from build123d import *

# Parameters (mm, degrees)
SKETCH1_R           = 1.2
BOSS_EXTRUDE1_DEPTH = 10
SKETCH3_R           = 13.5
SKETCH3_R_2         = 7.75
CUT_EXTRUDE1_DEPTH  = 1
SKETCH4_W           = 28.3
SKETCH4_H           = 8.75
CUT_EXTRUDE2_DEPTH  = 6.444
CUT_EXTRUDE3_DEPTH  = 0.1
CUT_EXTRUDE4_DEPTH  = 2


with BuildPart() as part:
    # Sketch1 → Boss-Extrude1 (new body)
    with BuildSketch(Plane(origin=(0, 0, 0), x_dir=(1, 0, 0), z_dir=(0, 1, 0))):
        with BuildLine():
            Line((-13.613846154, 16.730769231), (21.306153846, 16.730769231))
            ThreePointArc((21.306153846, 16.730769231), (23.10220507, 15.986820455), (23.846153846, 14.190769231))
            Line((23.846153846, 14.190769231), (23.846153846, -20.729230769))
            ThreePointArc((23.846153846, -20.729230769), (23.10220507, -22.525281993), (21.306153846, -23.269230769))
            Line((21.306153846, -23.269230769), (-13.613846154, -23.269230769))
            ThreePointArc((-13.613846154, -23.269230769), (-15.409897378, -22.525281993), (-16.153846154, -20.729230769))
            Line((-16.153846154, -20.729230769), (-16.153846154, 14.190769231))
            ThreePointArc((-16.153846154, 14.190769231), (-15.409897378, 15.986820455), (-13.613846154, 16.730769231))
        make_face()
        with Locations(Location((-13.613846154, 14.190769231, 0), (0, 0, 270))):
            Circle(SKETCH1_R, mode=Mode.SUBTRACT)
        with Locations(Location((21.386153846, 14.190769231, 0), (0, 0, 270))):
            Circle(SKETCH1_R, mode=Mode.SUBTRACT)
        with Locations(Location((21.386153846, -20.809230769, 0), (0, 0, 270))):
            Circle(SKETCH1_R, mode=Mode.SUBTRACT)
        with Locations(Location((-13.613846154, -20.809230769, 0), (0, 0, 270))):
            Circle(SKETCH1_R, mode=Mode.SUBTRACT)
    extrude(amount=BOSS_EXTRUDE1_DEPTH)

    # Sketch3 → Cut-Extrude1 (cut)
    with BuildSketch(Plane(origin=(0, 10, 0), x_dir=(1, 0, 0), z_dir=(0, 1, 0))):
        with Locations(Location((3.846153846, -7.269230769, 0), (0, 0, 270))):
            Circle(SKETCH3_R)
        with Locations(Location((3.846153846, -7.269230769, 0), (0, 0, 270))):
            Circle(SKETCH3_R_2, mode=Mode.SUBTRACT)
    extrude(amount=-CUT_EXTRUDE1_DEPTH, mode=Mode.SUBTRACT)

    # Sketch4 → Cut-Extrude2 (cut)
    with BuildSketch(Plane.ZY.offset(16.153846154)):
        with Locations((3.419230769, 5.092214042)):
            Rectangle(SKETCH4_W, SKETCH4_H)
    extrude(amount=-CUT_EXTRUDE2_DEPTH, mode=Mode.SUBTRACT)

    # Sketch5 → Cut-Extrude3 (cut)
    with BuildSketch(Plane(origin=(0, 10, 0), x_dir=(1, 0, 0), z_dir=(0, 1, 0))):
        Polygon((-12.625840765, 10.092905938), (-12.625840765, 8.58923838), (-8.593277769, 8.58923838), (-8.593277769, 7.290616398), (-12.625840765, 7.290616398), (-12.625840765, 5.771945506), (-15.223084728, 8.179147228), align=None)
    extrude(amount=-CUT_EXTRUDE3_DEPTH, mode=Mode.SUBTRACT)

    # Sketch6 → Cut-Extrude4 (cut)
    with BuildSketch(Plane.XZ):
        with BuildLine():
            Line((-16.153846154, 17.269230769), (-13.201846154, 17.269230769))
            ThreePointArc((-13.201846154, 17.269230769), (-11.046584685, 18.1619693), (-10.153846154, 20.317230769))
            Line((-10.153846154, 20.317230769), (-10.153846154, 23.269230769))
            Line((-10.153846154, 23.269230769), (-10.153846154, 27.06129419))
            Line((-10.153846154, 27.06129419), (-21.305262053, 27.06129419))
            Line((-21.305262053, 27.06129419), (-21.305262053, 17.269230769))
            Line((-21.305262053, 17.269230769), (-16.153846154, 17.269230769))
        make_face()
        with BuildLine():
            Line((23.846153846, 17.269230769), (20.894153846, 17.269230769))
            ThreePointArc((20.894153846, 17.269230769), (18.738892377, 18.1619693), (17.846153846, 20.317230769))
            Line((17.846153846, 20.317230769), (17.846153846, 23.269230769))
            Line((17.846153846, 23.269230769), (17.846153846, 27.06129419))
            Line((17.846153846, 27.06129419), (26.668789671, 27.06129419))
            Line((26.668789671, 27.06129419), (26.668789671, 17.269230769))
            Line((26.668789671, 17.269230769), (23.846153846, 17.269230769))
        make_face()
        with BuildLine():
            Line((-10.153846154, -16.730769231), (-10.153846154, -13.778769231))
            ThreePointArc((-10.153846154, -13.778769231), (-11.046584685, -11.623507762), (-13.201846154, -10.730769231))
            Line((-13.201846154, -10.730769231), (-16.153846154, -10.730769231))
            Line((-16.153846154, -10.730769231), (-21.305262053, -10.730769231))
            Line((-21.305262053, -10.730769231), (-21.305262053, -18.817505275))
            Line((-21.305262053, -18.817505275), (-10.153846154, -18.817505275))
            Line((-10.153846154, -18.817505275), (-10.153846154, -16.730769231))
        make_face()
        with BuildLine():
            Line((17.846153846, -16.730769231), (17.846153846, -13.778769231))
            ThreePointArc((17.846153846, -13.778769231), (18.738892377, -11.623507762), (20.894153846, -10.730769231))
            Line((20.894153846, -10.730769231), (23.846153846, -10.730769231))
            Line((23.846153846, -10.730769231), (26.668789671, -10.730769231))
            Line((26.668789671, -10.730769231), (26.668789671, -18.817505275))
            Line((26.668789671, -18.817505275), (17.846153846, -18.817505275))
            Line((17.846153846, -18.817505275), (17.846153846, -16.730769231))
        make_face()
    extrude(amount=-CUT_EXTRUDE4_DEPTH, mode=Mode.SUBTRACT)


solid = part.part
Here's how the part is built. I have some questions about the finished solid (model axes, mm). A direction names the side the tool comes from. Coordinates: 2 decimals unless noted, no trailing zeros. Write each loop counter-clockwise with the first axis right and the second up, starting at its lowest first coordinate (ties: lowest second). Pieces come first, ordered by that corner, then holes.
Item 1: If we mould it in two halves opening along Z, with no side actions, what happens to faces 1 (the flat face through (22, 1, 17.269)), 2 (the flat face through (20, 2, -14)), 3 (the cylindrical face through (-13.253, 5.944, 21.954)), 4 (the cylindrical face through (20.32, 5.94, -13.64))? For each: +Z half, -Z half, draft (parallel to the pull), parting line (faces both ways), or undercut.
Item 2: I want a section at A-A on y = 3.25. Write out the boundary of the cut face in (x, z).
Item 3: I want a section at D-D on z = 13. Write out the boundary of the cut face in (x, y), and give its area (3 significant figures).
Item 4: If I drill on line 1 (Y direction, x = -13.5, z = -1.5); line 2 (Z direction, x = -11, y = 3.25); line 3 (X direction, y = 9.5, z = 21.5), over which ranges is the centre line in solid material (lowest first)?
Item 5: On a 3-axis mill with a long thin cutter (end or side, diameter ignored), from which of +Z, -Z, +X, -X, +Y, -Y can I reach the whole of each face in a straight line? I mean faces 5 (the cylindrical face through (-11.02, 0.99, -11.65)), 6 (the cylindrical face through (18.8, 1, 18.1)), 7 (the flat face through (-13, 9.467, 3)), 8 (the flat face through (22, 1, -10.731)), 9 (the cylindrical face through (-10.724, 0.986, 18.542)). Say none if no direction works.
Item 6: I want a section at B-B on z = 18.5. Write out the boundary of the cut face in (x, y).
Item 7: I want a section at C-C on x = 2.5. Write out the boundary of the cut face in (y, z).
Item 8: Will these pins go through, and if not, where does the flat tip stop? pin 1 (1.7 mm diameter, centred on x = -12, z = 21.5, fed in from -Y); pin 2 (1 mm diameter, centred on x = 23, y = 1, fed in from +Z); pin 3 (0.8 mm diameter, centred on x = -15, y = 0, fed in from -Z); pin 4 (12 mm diameter, centred on x = 7.5, z = -10.5, fed in from -Y).
Findings below:
1. face 1: +Z half
1. face 2: draft
1. face 3: undercut
1. face 4: undercut
2. outline: (-16.15, -14.19) arc R2.54 ccw to (-13.61, -16.73) - (21.31, -16.73) arc R2.54 ccw to (23.85, -14.19) - (23.85, 20.73) arc R2.54 ccw to (21.31, 23.27) - (-13.61, 23.27) arc R2.54 ccw to (-16.15, 20.73) - (-16.15, 17.57) - (-9.71, 17.57) - (-9.71, -10.73) - (-16.15, -10.73) - close; hole circle Ø2.4 at (-13.61, -14.19); hole circle Ø2.4 at (-13.61, 20.81); hole circle Ø2.4 at (21.39, -14.19); hole circle Ø2.4 at (21.39, 20.81)
3. outline: (-16.15, 0) - (23.85, 0) - (23.85, 10) - (16.07, 10) - (16.07, 9) - (9.06, 9) - (9.06, 10) - (-1.37, 10) - (-1.37, 9) - (-8.38, 9) - (-8.38, 10) - (-16.15, 10) - (-16.15, 9.47) - (-9.71, 9.47) - (-9.71, 0.72) - (-16.15, 0.72) - close
3. area: 330 mm2
4. line 1: y = 0 to 0.72, 9.47 to 10
4. line 2: z = -16.73 to -10.73, 17.57 to 23.27
4. line 3: x = -16.03 to -14.6, -12.63 to 20.4, 22.37 to 23.73
5. face 5: -Z, -X, -Y
5. face 6: +Z, +X, -Y
5. face 7: -X
5. face 8: -Z, +X, -Y
5. face 9: +Z, -X, -Y
6. outline: (-16.15, 2) - (-10.75, 2) - (-10.75, 0) - (18.45, 0) - (18.45, 2) - (23.85, 2) - (23.85, 10) - (11.34, 10) - (11.34, 9) - (-3.65, 9) - (-3.65, 10) - (-16.15, 10) - close
7. outline: (0, -16.73) - (10, -16.73) - (10, -6.16) - (9, -6.16) - (9, -0.36) - (10, -0.36) - (10, 14.9) - (9, 14.9) - (9, 20.7) - (10, 20.7) - (10, 23.27) - (0, 23.27) - close
8. pin 1: stops at y = 2
8. pin 2: stops at z = 17.27
8. pin 3: stops at z = -10.73
8. pin 4: stops at y = 0
